from build123d import *

# Parameters (mm, degrees)
EXTRUDE_1_DEPTH     = 3
CUT_EXTRUDE_1_DEPTH = 10
EXTRUDE_START       = -3
EXTRUDE_2_DEPTH     = 3
SKETCH_4_R          = 1.75
CUT_EXTRUDE_2_DEPTH = 10
CUT_EXTRUDE_3_DEPTH = 10


with BuildPart() as part:
    # 草图1 → 凸台-拉伸1 (new body)
    with BuildSketch(Plane(origin=(0, 0, 0), x_dir=(1, 0, 0), z_dir=(0, 1, 0))):
        with BuildLine():
            Line((-66.78059141, 154.593992167), (66.78059141, 154.593992167))
            ThreePointArc((66.78059141, 154.593992167), (85.265515034, 148.222525736), (95.898700635, 131.814498742))
            Line((95.898700635, 131.814498742), (111.265547961, 69.844672358))
            ThreePointArc((111.265547961, 69.844672358), (112.147438737, 62.624165782), (111.265547961, 55.403659207))
            Line((111.265547961, 55.403659207), (95.898700635, -6.566167178))
            ThreePointArc((95.898700635, -6.566167178), (85.265515034, -22.974194171), (66.78059141, -29.345660602))
            Line((66.78059141, -29.345660602), (-66.78059141, -29.345660602))
            ThreePointArc((-66.78059141, -29.345660602), (-85.265515034, -22.974194171), (-95.898700635, -6.566167178))
            Line((-95.898700635, -6.566167178), (-111.265547961, 55.403659207))
            ThreePointArc((-111.265547961, 55.403659207), (-112.147438737, 62.624165782), (-111.265547961, 69.844672358))
            Line((-111.265547961, 69.844672358), (-95.898700635, 131.814498742))
            ThreePointArc((-95.898700635, 131.814498742), (-85.265515034, 148.222525736), (-66.78059141, 154.593992167))
        make_face()
    extrude(amount=EXTRUDE_1_DEPTH)

    # 草图2 → 切除-拉伸1 (cut)
    with BuildSketch(Plane.XZ):
        with BuildLine():
            Line((95.898700635, -131.814498742), (111.265547961, -69.844672358))
            ThreePointArc((111.265547961, -69.844672358), (112.145783913, -62.939263665), (111.410792816, -56.016888883))
            ThreePointArc((111.410792816, -56.016888883), (104.688448853, -60.381556842), (97.766986015, -56.340073582))
            ThreePointArc((97.766986015, -56.340073582), (0, 2.309946502), (-97.766986015, -56.340073582))
            ThreePointArc((-97.766986015, -56.340073582), (-104.688448853, -60.381556842), (-111.410792816, -56.016888883))
            ThreePointArc((-111.410792816, -56.016888883), (-112.145783913, -62.939263665), (-111.265547961, -69.844672358))
            Line((-111.265547961, -69.844672358), (-95.898700635, -131.814498742))
            ThreePointArc((-95.898700635, -131.814498742), (-85.265515034, -148.222525736), (-66.78059141, -154.593992167))
            Line((-66.78059141, -154.593992167), (66.78059141, -154.593992167))
            ThreePointArc((66.78059141, -154.593992167), (85.265515034, -148.222525736), (95.898700635, -131.814498742))
        make_face()
    extrude(amount=-CUT_EXTRUDE_1_DEPTH, mode=Mode.SUBTRACT)

    # 草图3 → 凸台-拉伸2 (add)
    with BuildSketch(Plane(origin=(0, 3, 0), x_dir=(1, 0, 0), z_dir=(0, 1, 0)).offset(EXTRUDE_START)):
        with BuildLine():
            Line((111.265547961, 55.403659207), (97.047161675, 55.012754554))
            ThreePointArc((97.047161675, 55.012754554), (100.513394998, 61.851126086), (103.498491265, 68.91280428))
            ThreePointArc((103.498491265, 68.91280428), (104.361855318, 69.927640036), (105.671102633, 70.174946664))
            ThreePointArc((105.671102633, 70.174946664), (110.30657274, 67.598027995), (112.147438737, 62.624165782))
            ThreePointArc((112.147438737, 62.624165782), (111.926149897, 58.98708431), (111.265547961, 55.403659207))
        make_face()
        with BuildLine():
            Line((-111.265547961, 55.403659207), (-97.047161675, 55.012754554))
            ThreePointArc((-97.047161675, 55.012754554), (-100.513394998, 61.851126086), (-103.498491265, 68.91280428))
            ThreePointArc((-103.498491265, 68.91280428), (-104.361855318, 69.927640036), (-105.671102633, 70.174946664))
            ThreePointArc((-105.671102633, 70.174946664), (-110.30657274, 67.598027995), (-112.147438737, 62.624165782))
            ThreePointArc((-112.147438737, 62.624165782), (-111.926149897, 58.98708431), (-111.265547961, 55.403659207))
        make_face()
    extrude(amount=EXTRUDE_2_DEPTH)

    # 草图4 → 切除-拉伸2 (cut)
    with BuildSketch(Plane(origin=(0, 3, 0), x_dir=(1, 0, 0), z_dir=(0, 1, 0))):
        with Locations(Location((104.507530951, 62.624165782, 0), (0, 0, 270))):
            Circle(SKETCH_4_R)
        with Locations(Location((-104.507530951, 62.624165782, 0), (0, 0, 270))):
            Circle(SKETCH_4_R)
        with Locations(Location((80.450184708, -16.818951307, 0), (0, 0, 270))):
            Circle(SKETCH_4_R)
        with Locations(Location((-80.450184708, -16.818951307, 0), (0, 0, 270))):
            Circle(SKETCH_4_R)
    extrude(amount=-CUT_EXTRUDE_2_DEPTH, mode=Mode.SUBTRACT)

    # 草图5 → 切除-拉伸3 (cut)
    with BuildSketch(Plane(origin=(0, 3, 0), x_dir=(1, 0, 0), z_dir=(0, 1, 0))):
        with BuildLine():
            Line((11.016648097, -20.513898252), (-11.016648097, -20.513898252))
            ThreePointArc((-11.016648097, -20.513898252), (-13.814702514, -21.911306641), (-14.378457093, -24.987674549))
            add(Edge.make_bspline(
                [(-14.378457093, -24.987674549), (-14.050661547, -26.11933694), (-10.489346867, -26.76009099), (-7.724749574, -26.493757466), (-5.904508816, -27.417302496), (-5.804576355, -27.473305111)],
                knots=[0, 0, 0, 0, 0.274123853, 0.745489655, 0.777393608, 0.777393608, 0.777393608, 0.777393608], degree=3))
            ThreePointArc((-5.804576355, -27.473305111), (-5.325885634, -28.59829127), (-6.293448421, -29.345660602))
            Line((-6.293448421, -29.345660602), (6.293448421, -29.345660602))
            ThreePointArc((6.293448421, -29.345660602), (5.325885634, -28.59829127), (5.804576355, -27.473305111))
            add(Edge.make_bspline(
                [(5.804576355, -27.473305111), (5.904508816, -27.417302496), (7.724749574, -26.493757466), (10.489346867, -26.76009099), (14.050661547, -26.11933694), (14.378457093, -24.987674549)],
                knots=[0, 0, 0, 0, 0.031903952, 0.503269754, 0.777393608, 0.777393608, 0.777393608, 0.777393608], degree=3))
            ThreePointArc((14.378457093, -24.987674549), (13.814702514, -21.911306641), (11.016648097, -20.513898252))
        make_face()
    extrude(amount=-CUT_EXTRUDE_3_DEPTH, mode=Mode.SUBTRACT)


solid = part.part
Part model, mm, in its own coordinate system. Coordinates: 2 decimals unless noted, no trailing zeros. Write each loop counter-clockwise with the first axis right and the second up, starting at its lowest first coordinate (ties: lowest second). Pieces come first, ordered by that corner, then holes. Notation, with made-up numbers: M 29.25,-19.5 L 53.25,-19.5 A25 cw 53.25,4.5 Z; hole C 14.25,-1.75 d9. An arc over 180 degrees is marked long. Return JSON: item names as keys, results as strings.
1. Saw through at A-A, the plane z = -51.5. Write the cut outline in (x, y), then the cut area to 3 significant figures.
Determined:
{"outline": "M -110.3,0 L -95.03,0 L -95.03,3 L -110.3,3 Z; M 95.03,0 L 110.3,0 L 110.3,3 L 95.03,3 Z", "area": "91.6 mm²"}
2. Saw through at D-D, the plane z = -29.5. Write the cut outline in (x, y), then the cut area to 3 significant figures.
Determined:
{"outline": "M -104.84,0 L -77.7,0 L -77.7,3 L -104.84,3 Z; M 77.7,0 L 104.84,0 L 104.84,3 L 77.7,3 Z", "area": "163 mm²"}
3. Probe L1, parallel to X at y = 1.95, z = -63.5; L2, parallel to X at y = 1.75, z = 17; L3, parallel to X at y = 0.9, z = -55. List the from-to ranges inside material, lowest first.
Determined:
{"L1": "-112.1 to -106.02, -102.99 to -101.26, 101.26 to 102.99, 106.02 to 112.1", "L2": "-91.04 to -82.19, -78.71 to 78.71, 82.19 to 91.04", "L3": "-111.17 to -97.04, 97.04 to 111.17"}
4. Saw through at C-C, the plane y = 1.55. Count the separate pieces of the cut face and the enclosed holes in it, then the cut area to 3 significant figures.
Determined:
{"separate pieces": "1", "enclosed holes": "4", "area": "8,940 mm²"}
5. Saw through at B-B, the plane x = 51. Write the cut outline in (y, z).
Determined:
{"outline": "M 0,-10.12 L 3,-10.12 L 3,29.35 L 0,29.35 Z"}
6. Flat gauge pins, fed straight in: pin 1 Ø1 at (y, z) = (0.5, 15.5) entering from +X; pin 2 Ø0.9 at (x, y) = (0.5, 1.5) entering from +Z. Where does each tip first touch, or does it go through?
Determined:
{"pin 1": "x = 92.37", "pin 2": "z = 20.51"}
